```python
from build123d import *

# Parameters (mm, degrees)
SKETCH2_R           = 40
SKETCH2_R_2         = 10
BOSS_EXTRUDE1_DEPTH = 12.5
SKETCH3_R           = 31.25
CUT_EXTRUDE1_DEPTH  = 10
SKETCH6_R           = 11
SKETCH6_R_2         = 10
BOSS_EXTRUDE2_DEPTH = 2
SKETCH4_R           = 3
CUT_EXTRUDE2_DEPTH  = 59.523499554
CIRPATTERN1_COUNT   = 5


with BuildPart() as part:
    # Sketch2 → Boss-Extrude1 (new, symmetric)
    with BuildSketch(Plane.XY):
        Circle(SKETCH2_R)
        Circle(SKETCH2_R_2, mode=Mode.SUBTRACT)
    extrude(amount=BOSS_EXTRUDE1_DEPTH, both=True)

    # Sketch3 → Cut-Extrude1 (cut)
    with BuildSketch(Plane.XY.offset(12.5)):
        Circle(SKETCH3_R)
    cut_extrude1 = extrude(amount=-CUT_EXTRUDE1_DEPTH, mode=Mode.SUBTRACT)

    # Sketch6 → Boss-Extrude2 (add)
    with BuildSketch(Plane.XY.offset(2.5)):
        Circle(SKETCH6_R)
        Circle(SKETCH6_R_2, mode=Mode.SUBTRACT)
    boss_extrude2 = extrude(amount=BOSS_EXTRUDE2_DEPTH)

    # Mirror1: Cut-Extrude1, Boss-Extrude2 across plane
    add(cut_extrude1.mirror(Plane.XY), mode=Mode.SUBTRACT)
    add(boss_extrude2.mirror(Plane.XY))

    # Sketch4 → Cut-Extrude2 (cut, through all)
    with BuildSketch(Plane.XY.offset(2.5)):
        with Locations((0, 17)):
            Circle(SKETCH4_R)
    cut_extrude2 = extrude(amount=-CUT_EXTRUDE2_DEPTH, mode=Mode.SUBTRACT)

    # CirPattern1: Cut-Extrude2 ×5 about axis
    cirpattern1_axis = Axis((0, 0, 0), (0, 0, 1))
    for i in range(1, CIRPATTERN1_COUNT):
        add(cut_extrude2.rotate(cirpattern1_axis, i * 360 / CIRPATTERN1_COUNT), mode=Mode.SUBTRACT)

    # Sketch5 → Cut-Revolve1 (revolve, cut)
    with BuildSketch(Plane(origin=(0, 0, 0), x_dir=(1, 0, 0), z_dir=(0, 1, 0)), mode=Mode.PRIVATE) as cut_revolve1_sk:
        Polygon((40, 9.5), (34, 6.035898385), (34, -6.035898385), (40, -9.5), align=None)
    revolve(cut_revolve1_sk.sketch.rotate(Axis((0, 0, -19.267509915), (0, 0, 1)), 180), axis=Axis((0, 0, -19.267509915), (0, 0, 1)), mode=Mode.SUBTRACT)


solid = part.part
```
CAD build for the part. Positions are in the model's coordinates, mm. A direction names the side the tool comes from. Round coordinates to 2 decimals unless told otherwise and drop trailing zeros. Order: outer loops, then holes, each group sorted by start corner. A loop starts at its lowest first (then second) coordinate and runs counter-clockwise, first axis right, second up. Notation, with made-up numbers: (88.5, 10) -> (135.5, 10) arc R30 cw to (135.5, 47) -> close; hole circle Ø9 at (49.25, -38.75). An arc over 180 degrees is marked (long way). Write item = value, one per line.
(1) Flat gauge pins, fed straight in: P1, Ø3, axis at x = -5, y = 16.5, coming from the -Z side; P2, Ø9.5, axis at x = 16.17, y = 5.25, coming from the +Z side; P3, Ø11, axis at x = -3.5, y = -4.5, coming from the -Z side. Where does each tip first touch, or does it go through?
Answers follow:
P1 = -2.5
P2 = 2.5
P3 = -4.5
(2) Cut at C-C (x = 0). State how many separate pieces and enclosed holes the cut face has, plus the area to 3 significant figures.
Answers follow:
separate_pieces = 3
enclosed_holes = 0
area = 442 mm²
(3) Cut at D-D (z = 0). Write the cut outline in (x, y), plus the area to 3 significant figures.
Answers follow:
outline = circle Ø68 at (0, 0); hole circle Ø6 at (-16.17, 5.25); hole circle Ø6 at (-9.99, -13.75); hole circle Ø20 at (0, 0); hole circle Ø6 at (0, 17); hole circle Ø6 at (9.99, -13.75); hole circle Ø6 at (16.17, 5.25)
area = 3,180 mm²
(4) Cut at B-B (z = -10.5). Write the cut outline in (x, y).
Answers follow:
outline = circle Ø80 at (0, 0); hole circle Ø62.5 at (0, 0)
(5) Drill centre lines: L1, parallel to Y at x = 0, z = 0.4; L2, parallel to Y at x = 7, z = -3.5; L3, parallel to X at y = 7, z = -2. Where is each one in solid material? Low to high.
Answers follow:
L1 = -34 to -10, 10 to 14, 20 to 34
L2 = -33.27 to -30.46, -8.49 to -7.14, 7.14 to 8.49, 30.46 to 33.27
L3 = -33.27 to -18.61, -13.73 to -7.14, 7.14 to 13.73, 18.61 to 33.27
(6) 3-axis set-ups, long thin cutter, end or side, ignore diameter. For faces 4 (the flat face through (2, -10, 4.5)), 5 (the conical face through (7.452, 33.558, 6.253)), 6 (the flat face through (2, -10, -4.5)): which of +Z, -Z, +X, -X, +Y, -Y reach the whole face in a straight line?
Answers follow:
face_4 = +Z
face_5 = none
face_6 = -Z
(7) Pull direction Y, two halves, no side cores. Call faces 1 (the cylindrical face through (-8.67, -39.05, -10.98)), 2 (the flat face through (-24, -21, -12.5)), 3 (the cylindrical face through (-31.22, 1.37, 7.57)): +Y half, -Y half, draft (parallel to the pull), parting line (faces both ways), or undercut.
Answers follow:
face_1 = parting line
face_2 = draft
face_3 = undercut
